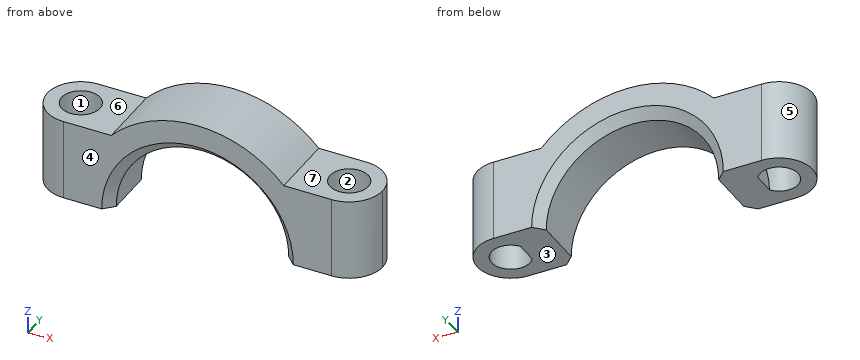
from build123d import *

# Parameters (mm, degrees)
CROQUIS1_R                = 2
SALIENTE_EXTRUIR1_DEPTH   = 8.5
SALIENTE_EXTRUIR1_2_DEPTH = 8.5
SALIENTE_EXTRUIR2_DEPTH   = 7
CHAFL_N1_SIZE             = 1


with BuildPart() as part:
    # Croquis1 → Saliente-Extruir1 (new body)
    with BuildSketch(Plane.XY):
        with BuildLine():
            Line((23, 3.5), (23, -3.5))
            Line((23, -3.5), (28, -3.5))
            ThreePointArc((28, -3.5), (30.474873734, -2.474873734), (31.5, 0))
            ThreePointArc((31.5, 0), (30.474873734, 2.474873734), (28, 3.5))
            Line((28, 3.5), (23, 3.5))
        make_face()
        with Locations((28, 0)):
            Circle(CROQUIS1_R, mode=Mode.SUBTRACT)
    extrude(amount=SALIENTE_EXTRUIR1_DEPTH)



with BuildPart() as body_2:
    # Croquis1 → Saliente-Extruir1 2 (new body)
    with BuildSketch(Plane.XY):
        with BuildLine():
            Line((5, -3.5), (5, 3.5))
            Line((5, 3.5), (0, 3.5))
            ThreePointArc((0, 3.5), (-3.5, 0), (0, -3.5))
            Line((0, -3.5), (5, -3.5))
        make_face()
        Circle(CROQUIS1_R, mode=Mode.SUBTRACT)
    extrude(amount=SALIENTE_EXTRUIR1_2_DEPTH)


with BuildPart() as part_1:
    add(part.part)

    add(body_2.part)  # Saliente-Extruir2 merges body 2
    # Croquis2 → Saliente-Extruir2 (add, through all)
    with BuildSketch(Plane.XZ.offset(3.5)):
        with BuildLine():
            Line((1.620581602, 2e-09), (5.000000002, 2e-09))
            ThreePointArc((5.000000002, 2e-09), (14.000000002, 9.000000002), (23.000000002, 2e-09))
            Line((23.000000002, 2e-09), (26.379418402, 2e-09))
            ThreePointArc((26.379418402, 2e-09), (14.000000002, 12.379418402), (1.620581602, 2e-09))
        make_face()
    extrude(amount=-SALIENTE_EXTRUIR2_DEPTH)

    # Chaflán1
    chafl_n1_edges = [part_1.edges().sort_by_distance(p)[0] for p in [
        (14.000000002, 3.5, 9.000000002),
        (14.000000002, -3.5, 9.000000002),
    ]]
    chamfer(chafl_n1_edges, length=CHAFL_N1_SIZE)


solid = part_1.part
Verification items for the finished model (mm, model axes). Face numbers are marked on the shaded views. A direction names the side the tool comes from. Coordinates: 2 decimals unless noted, no trailing zeros. Order: outer loops, then holes, each group sorted by start corner. A loop starts at its lowest first (then second) coordinate and runs counter-clockwise, first axis right, second up. Notation, with made-up numbers: M 8,84 L 37,84 A19 ccw 37,102 Z; hole C -35,76 d3. An arc over 180 degrees is marked long. One line per item, written item: value. Start each with the question number.
Item 1: Thickness scan on probe 1 along X at (y, z) = (-1.75, 2); probe 2 along X at (y, z) = (-0.5, 5.5); probe 3 along Y at (x, z) = (1, 2.5). Record the ranges inside material, lowest first.
Item 2: Depth check by flat-ended pin: P1, Ø2, axis at y = -1.5, z = 7.5, coming from the +X side; P2, Ø3, axis at x = 16.5, y = 1.5, coming from the +Z side. Enter the tip coordinate at first touch or a pass-through.
Item 3: Sectioned sample at A-A on y = -1.5. Record the cut outline in (x, z).
Item 4: Mould release check, pull along Y, two halves, no side actions. Record for the marked faces 1, 2, 3 and 4: pulls with the +Y half, pulls with the -Y half, needs draft (parallel to the pull), parting line crosses it, or undercut.
Item 5: Sectioned sample at B-B on x = 25. Record the cut outline in (y, z).
Item 6: Sectioned sample at C-C on z = 4.75. Give the number of separate pieces and of enclosed holes in the cut face, then the cut area to 3 significant figures.
Item 7: Access from +Z, -Z, +X, -X, +Y, -Y to the whole of each face (thin tool, end or side, straight path). Record for the marked faces 5, 6 and 7.
Calculated:
1. probe 1: -3.03 to -0.97, 0.97 to 5.23, 22.77 to 27.03, 28.97 to 31.03
1. probe 2: -3.46 to -1.94, 1.94 to 6.88, 21.12 to 26.06, 29.94 to 31.46
1. probe 3: -3.5 to -1.73, 1.73 to 3.5
2. P1: x = 31.46
2. P2: z = 12.34
3. outline: M -3.16,0 L -1.32,0 L -1.32,8.5 L -3.16,8.5 Z; M 1.32,0 L 5,0 A9 cw 23,0 L 26.68,0 L 26.68,8.5 L 23,8.5 A12.38 ccw 5,8.5 L 1.32,8.5 Z; M 29.32,0 L 31.16,0 L 31.16,8.5 L 29.32,8.5 Z
4. face 1: undercut
4. face 2: undercut
4. face 3: needs draft
4. face 4: pulls with the -Y half
5. outline: M -3.5,0 L 3.5,0 L 3.5,8.5 L -3.5,8.5 Z
6. separate pieces: 2
6. enclosed holes: 2
6. area: 100 mm^2
7. face 5: +Z, -Z, -X
7. face 6: +Z, -X, +Y, -Y
7. face 7: +Z, +X, +Y, -Y
